from build123d import *

# Parameters (mm, degrees)
SKETCH1_R           = 37
BOSS_EXTRUDE1_DEPTH = 28.25
SKETCH2_R           = 28.8
CUT_EXTRUDE1_DEPTH  = 11
SKETCH3_R           = 22.5
CUT_EXTRUDE2_DEPTH  = 8.75
SKETCH4_R           = 21.05
CUT_EXTRUDE3_DEPTH  = 7
SKETCH5_R           = 19.5
CUT_EXTRUDE4_DEPTH  = 59.767018812
SKETCH6_R           = 1.675
CUT_EXTRUDE5_DEPTH  = 15.75
CIRPATTERN1_COUNT   = 11
SKETCH7_R           = 1.7
CUT_EXTRUDE6_DEPTH  = 60.464800513
SKETCH8_R           = 3.1
CUT_EXTRUDE7_DEPTH  = 16.75


with BuildPart() as part:
    # Sketch1 → Boss-Extrude1 (new body)
    with BuildSketch(Plane(origin=(0, 0, 0), x_dir=(1, 0, 0), z_dir=(0, 1, 0))):
        with Locations(Location((0, 0, 0), (0, 0, 270))):
            Circle(SKETCH1_R)
    extrude(amount=BOSS_EXTRUDE1_DEPTH)

    # Sketch2 → Cut-Extrude1 (cut)
    with BuildSketch(Plane(origin=(0, 0, 0), x_dir=(1, 0, 0), z_dir=(0, 1, 0))):
        with Locations(Location((0, 0, 0), (0, 0, 270))):
            Circle(SKETCH2_R)
    extrude(amount=CUT_EXTRUDE1_DEPTH, mode=Mode.SUBTRACT)

    # Sketch3 → Cut-Extrude2 (cut)
    with BuildSketch(Plane.XZ.offset(-11)):
        with Locations(Location((0, 0, 0), (0, 0, 270))):
            Circle(SKETCH3_R)
    extrude(amount=-CUT_EXTRUDE2_DEPTH, mode=Mode.SUBTRACT)

    # Sketch4 → Cut-Extrude3 (cut)
    with BuildSketch(Plane.XZ.offset(-19.75)):
        with Locations(Location((0, 0, 0), (0, 0, 270))):
            Circle(SKETCH4_R)
    extrude(amount=-CUT_EXTRUDE3_DEPTH, mode=Mode.SUBTRACT)

    # Sketch5 → Cut-Extrude4 (cut, through all)
    with BuildSketch(Plane.XZ.offset(-26.75)):
        with Locations(Location((0, 0, 0), (0, 0, 270))):
            Circle(SKETCH5_R)
    extrude(amount=-CUT_EXTRUDE4_DEPTH, mode=Mode.SUBTRACT)

    # Sketch6 → Cut-Extrude5 (cut)
    with BuildSketch(Plane(origin=(0, 0, 0), x_dir=(1, 0, 0), z_dir=(0, 1, 0))):
        with Locations(Location((27, 0, 0), (0, 0, 270))):
            Circle(SKETCH6_R)
    cut_extrude5 = extrude(amount=CUT_EXTRUDE5_DEPTH, mode=Mode.SUBTRACT)

    # CirPattern1: Cut-Extrude5 ×11 about axis
    cirpattern1_axis = Axis((0, 0, 0), (0, 1, 0))
    for i in range(1, CIRPATTERN1_COUNT):
        add(cut_extrude5.rotate(cirpattern1_axis, i * 360 / CIRPATTERN1_COUNT), mode=Mode.SUBTRACT)

    # Sketch7 → Cut-Extrude6 (cut, through all)
    with BuildSketch(Plane(origin=(0, 0, 0), x_dir=(1, 0, 0), z_dir=(0, 1, 0))):
        with Locations(Location((31.184102699, 9.154328969, 0), (0, 0, 270))):
            Circle(SKETCH7_R)
        with Locations(Location((-13.503333209, 29.56196868, 0), (0, 0, 270))):
            Circle(SKETCH7_R)
        with Locations(Location((-32.5, 0, 0), (0, 0, 270))):
            Circle(SKETCH7_R)
        with Locations(Location((4.624211408, -32.169343619, 0), (0, 0, 270))):
            Circle(SKETCH7_R)
    extrude(amount=CUT_EXTRUDE6_DEPTH, mode=Mode.SUBTRACT)

    # Sketch8 → Cut-Extrude7 (cut)
    with BuildSketch(Plane(origin=(0, 28.25, 0), x_dir=(1, 0, 0), z_dir=(0, 1, 0))):
        with Locations(Location((31.184102699, 9.154328969, 0), (0, 0, 270))):
            Circle(SKETCH8_R)
        with Locations(Location((-13.503333209, 29.56196868, 0), (0, 0, 270))):
            Circle(SKETCH8_R)
        with Locations(Location((-32.5, 0, 0), (0, 0, 270))):
            Circle(SKETCH8_R)
        with Locations(Location((4.624211408, -32.169343619, 0), (0, 0, 270))):
            Circle(SKETCH8_R)
    extrude(amount=-CUT_EXTRUDE7_DEPTH, mode=Mode.SUBTRACT)


solid = part.part
Build history of the part. All positions in model axes, mm. A direction names the side the tool comes from. Give positions to 0.01 mm unless a question says otherwise; leave off trailing zeros. Write each loop counter-clockwise with the first axis right and the second up, starting at its lowest first coordinate (ties: lowest second). Pieces come first, ordered by that corner, then holes. Notation, with made-up numbers: (-10, 60.5) - (2, 60.5) arc R29 ccw to (2, 84.5) - close; hole circle Ø2 at (13.5, 39.25). An arc over 180 degrees is marked (long way). Use one line per item in the form item = value. Start each with the question number.
1. Two-plate mould, pull along Z, no slides. Class faces 1 (the face through (-15, 11.5, -28)), 2 (the face through (8, 0, -28)): released by +Z, released by -Z, zero draft, split by the parting line, or undercut.
2. Band-saw the part on A-A on x = 0. Write the cut outline in (y, z), plus the area to 3 significant figures.
3. Band-saw the part on B-B on z = 0. Count the separate pieces of the cut face and the enclosed holes in it, plus the area to 3 significant figures.
4. Drop flat-ended pins along their axis: pin 1 Ø3 at (x, y) = (-7, 13.5) entering from +Z; pin 2 Ø8 at (x, y) = (-24, 5.5) entering from +Z; pin 3 Ø2 at (x, y) = (1.5, 25) entering from -Z; pin 4 Ø2 at (x, z) = (-13.5, -29.56) entering from -Y. Give the stop position or say it passes through.
5. Band-saw the part on D-D on x = 27. Write the cut outline in (y, z) (3 decimals), plus the area to 3 significant figures.
6. 3-axis set-ups, long thin cutter, end or side, ignore diameter. For faces 3 (the face through (25.365, 13.342, -0.363)), 4 (the face through (19.334, 27.49, 2.539)), 5 (the face through (34.258, 19.992, -9.558)): which of +Z, -Z, +X, -X, +Y, -Y reach the whole face in a straight line?
7. Probe line 1 (X direction, y = 25, z = 0); line 2 (X direction, y = 7.25, z = 0); line 3 (Z direction, x = 7, y = 14.5). List the from-to ranges inside material, lowest first. Write a range as [from, to].
Conclusion:
q1.face_1 = undercut
q1.face_2 = zero draft
q2.outline = (0, -37) - (28.25, -37) - (28.25, -19.5) - (26.75, -19.5) - (26.75, -21.05) - (19.75, -21.05) - (19.75, -22.5) - (11, -22.5) - (11, -28.8) - (0, -28.8) - close; (0, 28.8) - (11, 28.8) - (11, 22.5) - (19.75, 22.5) - (19.75, 21.05) - (26.75, 21.05) - (26.75, 19.5) - (28.25, 19.5) - (28.25, 37) - (0, 37) - close
q2.area = 710 mm²
q3.separate_pieces = 3
q3.enclosed_holes = 0
q3.area = 551 mm²
q4.pin_1 = 36.59
q4.pin_2 = 31.13
q4.pin_3 = -37
q4.pin_4 = through
q5.outline = (0, -25.298) - (28.25, -25.298) - (28.25, 25.298) - (0, 25.298) - (0, 10.022) - (11, 10.022) - (11, 1.675) - (15.75, 1.675) - (15.75, -1.675) - (11, -1.675) - (11, -10.022) - (0, -10.022) - close
q5.area = 1,190 mm²
q6.face_3 = -Y
q6.face_4 = +Y, -Y
q6.face_5 = +Y
q7.line_1 = [-37, -35.6], [-29.4, -21.05], [21.05, 37]
q7.line_2 = [-37, -34.2], [-30.8, -28.8], [28.8, 37]
q7.line_3 = [-36.33, -21.38], [21.38, 30.18], [34.16, 36.33]
